from build123d import *

# Parameters (mm, degrees)
F0_W     = 127
F0_H     = 76.2
F2_DEPTH = 5.969
F3_R     = 2.032
F4_DEPTH = 5.969


# Not quite as in the source:
# - a variable given as a bare number and used for a length is read in inches; the dataset says mm whatever the document's units were


with BuildPart() as f2:
    # F0 (on Top) → F2 (new body)
    with BuildSketch(Plane.XY):
        Rectangle(F0_W, F0_H)
    extrude(amount=F2_DEPTH)

    # F3 (on face) → F4 (cut, through all)
    with BuildSketch(Plane.XY.offset(5.969)):
        with BuildLine():
            ThreePointArc((-39.4335, -29.9085), (-40.0286590206, -28.4716590206), (-41.4655, -27.8765))
            ThreePointArc((-41.4655, -27.8765), (-42.9023409794, -31.3453409794), (-39.4335, -29.9085))
        make_face()
        with BuildLine():
            ThreePointArc((-17.018, -29.9085), (-17.6131590206, -28.4716590206), (-19.05, -27.8765))
            ThreePointArc((-19.05, -27.8765), (-20.4868409794, -31.3453409794), (-17.018, -29.9085))
        make_face()
        with BuildLine():
            Line((6.35, 0), (4.318, 0))
            ThreePointArc((4.318, 0), (6.35, -2.032), (8.382, 0))
            Line((8.382, 0), (6.35, 0))
        make_face()
        with BuildLine():
            ThreePointArc((8.382, 0), (6.35, 2.032), (4.318, 0))
            Line((4.318, 0), (6.35, 0))
            Line((6.35, 0), (8.382, 0))
        make_face()
        with BuildLine():
            ThreePointArc((27.432, -25.4), (26.8368409794, -23.9631590206), (25.4, -23.368))
            ThreePointArc((25.4, -23.368), (23.9631590206, -26.8368409794), (27.432, -25.4))
        make_face()
        with Locations((-41.4655, 29.9085)):
            Circle(F3_R)
        with Locations((-19.05, 29.9085)):
            Circle(F3_R)
        with Locations((25.4, 25.4)):
            Circle(F3_R)
    extrude(amount=-F4_DEPTH, mode=Mode.SUBTRACT)


solid = f2.part
For this review, take the finished solid that the model builds, in its own axes (mm). Round coordinates to 2 decimals unless told otherwise and drop trailing zeros. Order: outer loops, then holes, each group sorted by start corner. A loop starts at its lowest first (then second) coordinate and runs counter-clockwise, first axis right, second up. Notation, with made-up numbers: M 20.5,-13.75 L 34.5,-13.75 A22 cw 34.5,17.25 Z; hole C -28.5,-37 d10. An arc over 180 degrees is marked long. Write each question's results on one line, items separated by ' | '. Start each with the question number.
1. Clearance check with flat-ended pins moving along their axes: pin 1 Ø3.5 at (x, y) = (25.4, 25.4) entering from -Z; pin 2 Ø8 at (x, y) = (32.5, -5.5) entering from -Z. State where each tip first meets the part, or that it passes through.
2. Add section B-B (x = 6.35). State the section outline as (y, z) points, then the cut area to 3 significant figures.
3. Draft analysis for pull direction X (two halves, no side actions). For faces 1 (the face through (-1, 1, 5.969)), 2 (the face through (63.5, -1, 3)), 3 (the face through (-19.315, 31.923, 3.026)), state which applies: pulls with the +X half, pulls with the -X half, needs draft (parallel to the pull), parting line crosses it, or undercut.
4. To check wall thickness, follow L1, parallel to Y at x = -19.05, z = 4.25; L2, parallel to X at y = -25.4, z = 3.25. State the ranges of each line that lie inside material, in increasing order. Write a range as [from, to].
5. Add section A-A (y = 25.4). State the section outline as (x, z) points, then the cut area to 3 significant figures.
Output values:
1) pin 1: through | pin 2: z = 0
2) outline: M -38.1,0 L -2.03,0 L -2.03,5.97 L -38.1,5.97 Z; M 2.03,0 L 38.1,0 L 38.1,5.97 L 2.03,5.97 Z | area: 431 mm^2
3) face 1: needs draft | face 2: pulls with the +X half | face 3: undercut
4) L1: [-38.1, -31.94], [-27.88, 27.88], [31.94, 38.1] | L2: [-63.5, 23.37], [27.43, 63.5]
5) outline: M -63.5,0 L 23.37,0 L 23.37,5.97 L -63.5,5.97 Z; M 27.43,0 L 63.5,0 L 63.5,5.97 L 27.43,5.97 Z | area: 734 mm^2
